```python
from build123d import *

# Parameters (mm, degrees)
F0_W     = 12.7
F0_H     = 25.4
F1_DEPTH = 25.4
F2_W     = 12.7
F2_H     = 12.7
F3_DEPTH = 6.35
F4_W     = 12.7
F4_H     = 25.4
F5_DEPTH = 25.4
F7_DEPTH = 12.701
F8_R     = 6.35
F9_DEPTH = 12.701


with BuildPart() as f1:
    # F0 (on Front) → F1 (new body)
    with BuildSketch(Plane.XZ):
        with Locations((6.35, -12.7)):
            Rectangle(F0_W, F0_H)
    extrude(amount=F1_DEPTH)

    # F2 (on face) → F3 (cut)
    with BuildSketch(Plane.XZ.offset(25.4)):
        with Locations((6.35, -12.7)):
            Rectangle(F2_W, F2_H)
    extrude(amount=-F3_DEPTH, mode=Mode.SUBTRACT)

    # F4 (on face) → F5 (join)
    with BuildSketch(Plane.YZ.offset(12.7)):
        with Locations((-6.35, -12.7)):
            Rectangle(F4_W, F4_H)
    extrude(amount=F5_DEPTH)

    # F6 (on face) → F7 (cut, through all)
    with BuildSketch(Plane.XZ.offset(12.7)):
        with BuildLine():
            ThreePointArc((38.1, -12.7), (36.424032, -19.799516), (31.75, -25.4))
            Line((31.75, -25.4), (38.1, -25.4))
            Line((38.1, -25.4), (38.1, -12.7))
        make_face()
        with BuildLine():
            ThreePointArc((31.75, 0), (36.424032, -5.600484), (38.1, -12.7))
            Line((38.1, -12.7), (38.1, 0))
            Line((38.1, 0), (31.75, 0))
        make_face()
    extrude(amount=-F7_DEPTH, mode=Mode.SUBTRACT)

    # F8 (on face) → F9 (cut, through all)
    with BuildSketch(Plane.XZ.offset(12.7)):
        with Locations((25.4, -12.7)):
            Circle(F8_R)
    extrude(amount=-F9_DEPTH, mode=Mode.SUBTRACT)


solid = f1.part
```
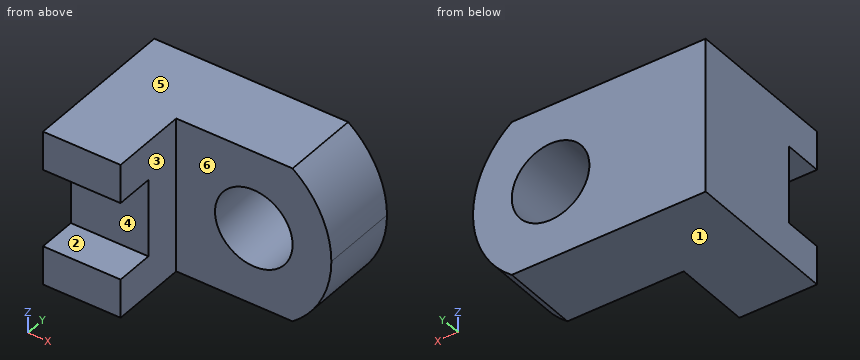
Can you work these out from the model? Positions are in its coordinate system, mm. Face numbers are marked on the shaded views. A direction names the side the tool comes from. Give positions to 0.01 mm unless a question says otherwise; leave off trailing zeros. Loops run counter-clockwise (first coordinate to the right, second up) from the corner with the lowest first, then second, coordinate; pieces in that order, holes last. Notation, with made-up numbers: M -34,-17.5 L -7,-17.5 A11 cw -7,-4.5 Z; hole C 2.25,56 d2. An arc over 180 degrees is marked long. One line per question, with ' | ' between items. Start each with the question number.
Q1. If we section it at A-A (x = 25.4): Please give me the cut outline in (y, z), plus the area to 3 significant figures.
Q2. For the marked faces 1, 2 and 3, which set-ups out of +Z, -Z, +X, -X, +Y, -Y let a thin tool reach every point of the face, with its end or its side?
Q3. If we section it at C-C (y = -5.5): Please give me the cut outline in (x, z) (3 decimals), plus the area to 4 significant figures.
Q4. If I drill on line 1 (Z direction, x = 25.4, y = -8); line 2 (Y direction, x = 32.5, z = -7); line 3 (Z direction, x = 21, y = -8.5), over which ranges is the centre line in solid material (lowest first)? Write a range as from..to.
Q5. For pin 1 Ø4 at (y, z) = (-16, -12.5) entering from +X; pin 2 Ø2 at (y, z) = (-7, -17.5) entering from +X; pin 3 Ø5 at (y, z) = (-14.5, -3) entering from +X, each with a flat end and sliding along its axis, tell me the tip position at first contact or that it passes through.
Q6. If we mould it in two halves opening along Z, with no side actions, what happens to the marked faces 4, 5 and 6? For each: +Z half, -Z half, draft (parallel to the pull), parting line (faces both ways), or undercut.
Q7. If we section it at B-B (z = -11.25): Please give me the cut outline in (x, y), plus the area to 3 significant figures.
Q8. If we section it at D-D (y = -15.75): Please give me the cut outline in (x, z), plus the area to 3 significant figures.
Computed:
1) outline: M -12.7,-25.4 L 0,-25.4 L 0,-19.05 L -12.7,-19.05 Z; M -12.7,-6.35 L 0,-6.35 L 0,0 L -12.7,0 Z | area: 161 mm²
2) face 1: -Z, +X, -X, +Y, -Y | face 2: +X, -X, -Y | face 3: +Z, -Z, +X, -Y
3) outline: M 0,-25.4 L 31.75,-25.4 A15.875 ccw 38.1,-12.7 A15.875 ccw 31.75,0 L 0,0 Z; hole C 25.4,-12.7 d12.7 | area: 792.5 mm²
4) line 1: z = -25.4..-19.05, -6.35..0 | line 2: y = -12.7..0 | line 3: z = -25.4..-17.28, -8.12..0
5) pin 1: stops at x = 12.7 | pin 2: stops at x = 37.64 | pin 3: stops at x = 35.96
6) face 4: undercut | face 5: +Z half | face 6: draft
7) outline: M 0,-19.05 L 12.7,-19.05 L 12.7,-12.7 L 19.22,-12.7 L 19.22,0 L 0,0 Z; M 31.58,-12.7 L 38.03,-12.7 L 38.03,0 L 31.58,0 Z | area: 407 mm²
8) outline: M 0,-25.4 L 12.7,-25.4 L 12.7,0 L 0,0 Z | area: 323 mm²
